Source: CAD feature listing. Evaluate the final solid. Frame: model axes, mm. Face numbers are marked on the shaded views. A direction names the side the tool comes from. Give positions to 0.01 mm unless a question says otherwise; leave off trailing zeros. Order: outer loops, then holes, each group sorted by start corner. A loop starts at its lowest first (then second) coordinate and runs counter-clockwise, first axis right, second up. Notation, with made-up numbers: M 66,63.5 L 116,63.5 A14 cw 116,67.5 Z; hole C 72.5,75.25 d8. An arc over 180 degrees is marked long. Answer in a Markdown table with one row per item. Add a question column.
(1) Section query B-B, the plane y = 7. Return loops of the section in (x, z) (3 decimals).
(2) Set-up query: the marked faces 1 and 2. Return all of +Z, -Z, +X, -X, +Y, -Y with unobstructed straight access to the full face (end or side cutting, diameter ignored); none if empty.
(3) Section query D-D, the plane x = -7. Return loops of the section in (y, z).
(4) Material intervals for line 1 along Y through (x, z) = (21.5, 10.5); line 2 along X through (y, z) = (2.5, 15); line 3 along X through (y, z) = (-22.5, 20.75), sorted ascending.
(5) Section query A-A, the plane z = 16.5. Return loops of the section in (x, y), plus the area to 3 significant figures.
(6) Mould query, pull axis Y, two halves, no side actions, for the marked faces 3, 4 and 5. Classes: pulls with the +Y half, pulls with the -Y half, needs draft (parallel to the pull), parting line crosses it, or undercut.
(7) Section query C-C, the plane z = 9.5. Return loops of the section in (x, y).
(8) Pin query (flat end, axial travel): P1, Ø3, axis at x = 27, y = -17, coming from the +Z side; P2, Ø3.5, axis at x = 33.25, y = 23.25, coming from the +Z side; P3, Ø1.2, axis at x = 36, z = 8, coming from the +Y side; P4, Ø2.5, axis at x = 27.4, y = 17.4, coming from the +Z side. Return the tip coordinate at first contact, or that it passes through.
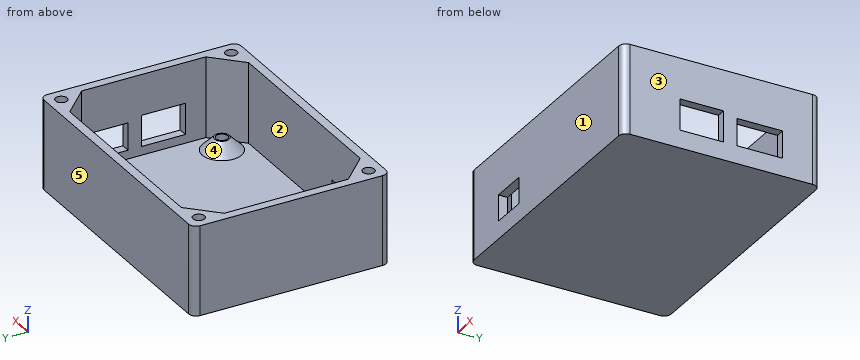
from build123d import *

# Parameters (mm, degrees)
SKETCH5_W           = 74
SKETCH5_H           = 54
BOSS_EXTRUDE4_DEPTH = 24.5
SHELL1_T            = -2.5
SKETCH6_R           = 2
BOSS_EXTRUDE5_DEPTH = 3.4
SKETCH11_R          = 1.6
CUT_EXTRUDE2_DEPTH  = 4.5
CUT_EXTRUDE4_REACH  = 84.494
SKETCH12_W          = 7.45
SKETCH12_H          = 12.5
CUT_EXTRUDE5_REACH  = 84.494
SKETCH13_W          = 8.5
SKETCH13_H          = 12
CUT_EXTRUDE6_REACH  = 71.895
SKETCH14_W          = 10
SKETCH14_H          = 7.138154435
BOSS_EXTRUDE7_DEPTH = 22
SKETCH9_R           = 1.6
CUT_EXTRUDE1_DEPTH  = 6.1
CHAMFER10_SIZE      = 3.4
CHAMFER11_SIZE      = 3.4
FILLET1_R           = 2


with BuildPart() as part:
    # Sketch5 → Boss-Extrude4 (new body)
    with BuildSketch(Plane.XY):
        Rectangle(SKETCH5_W, SKETCH5_H)
    extrude(amount=BOSS_EXTRUDE4_DEPTH)

    # Shell1
    shell1_openings = [part.faces().sort_by_distance(p)[0] for p in [
        (0, 0, 24.5),
    ]]
    offset(amount=SHELL1_T, openings=shell1_openings, kind=Kind.INTERSECTION)

    # Sketch6 → Boss-Extrude5 (add)
    with BuildSketch(Plane.XY.offset(2.5)):
        with Locations((-27.4, 17.4)):
            Circle(SKETCH6_R)
        with Locations((27.4, 17.4)):
            Circle(SKETCH6_R)
        with Locations((27.4, -17.4)):
            Circle(SKETCH6_R)
        with Locations((-27.4, -17.4)):
            Circle(SKETCH6_R)
    extrude(amount=BOSS_EXTRUDE5_DEPTH)

    # Sketch11 → Cut-Extrude2 (cut)
    with BuildSketch(Plane.XY.offset(5.9)):
        with Locations((-27.4, 17.4)):
            Circle(SKETCH11_R)
        with Locations((27.4, 17.4)):
            Circle(SKETCH11_R)
        with Locations((-27.4, -17.4)):
            Circle(SKETCH11_R)
        with Locations((27.4, -17.4)):
            Circle(SKETCH11_R)
    extrude(amount=-CUT_EXTRUDE2_DEPTH, mode=Mode.SUBTRACT)

    # Sketch12 → Cut-Extrude4 (cut, up to next)
    with BuildSketch(Plane(origin=(37, 0, 0), x_dir=(0, 0, -1), z_dir=(1, 0, 0)), mode=Mode.PRIVATE) as cut_extrude4_sk1:
        with Locations((-8.6, 10.53)):
            Rectangle(SKETCH12_W, SKETCH12_H)
    cut_extrude4_tool1 = extrude(cut_extrude4_sk1.sketch, amount=-CUT_EXTRUDE4_REACH, mode=Mode.PRIVATE) & part.part
    add(cut_extrude4_tool1.solids().sort_by_distance((37, 10.53, 8.6))[0], mode=Mode.SUBTRACT)

    # Sketch13 → Cut-Extrude5 (cut, up to next)
    with BuildSketch(Plane(origin=(37, 0, 0), x_dir=(0, 0, -1), z_dir=(1, 0, 0)), mode=Mode.PRIVATE) as cut_extrude5_sk1:
        with Locations((-9.125, -5.4)):
            Rectangle(SKETCH13_W, SKETCH13_H)
    cut_extrude5_tool1 = extrude(cut_extrude5_sk1.sketch, amount=-CUT_EXTRUDE5_REACH, mode=Mode.PRIVATE) & part.part
    add(cut_extrude5_tool1.solids().sort_by_distance((37, -5.4, 9.125))[0], mode=Mode.SUBTRACT)

    # Sketch14 → Cut-Extrude6 (cut, up to next)
    with BuildSketch(Plane.XZ.offset(27), mode=Mode.PRIVATE) as cut_extrude6_sk1:
        with Locations((-18.22, 8.449077218)):
            Rectangle(SKETCH14_W, SKETCH14_H)
    cut_extrude6_tool1 = extrude(cut_extrude6_sk1.sketch, amount=-CUT_EXTRUDE6_REACH, mode=Mode.PRIVATE) & part.part
    add(cut_extrude6_tool1.solids().sort_by_distance((-18.22, -27, 8.449077))[0], mode=Mode.SUBTRACT)

    # Sketch7 → Boss-Extrude7 (add)
    with BuildSketch(Plane.XY.offset(2.5)):
        Polygon((-27, 24.5), (-34.5, 17), (-34.5, 24.5), align=None)
        Polygon((-34.5, -17), (-27, -24.5), (-34.5, -24.5), align=None)
        Polygon((27, -24.5), (34.5, -17), (34.5, -24.5), align=None)
        Polygon((34.5, 17), (27, 24.5), (34.5, 24.5), align=None)
    extrude(amount=BOSS_EXTRUDE7_DEPTH)

    # Sketch9 → Cut-Extrude1 (cut)
    with BuildSketch(Plane.XY.offset(24.5)):
        with Locations((-33.25, 23.25)):
            Circle(SKETCH9_R)
        with Locations((33.25, 23.25)):
            Circle(SKETCH9_R)
        with Locations((-33.25, -23.25)):
            Circle(SKETCH9_R)
        with Locations((33.25, -23.25)):
            Circle(SKETCH9_R)
    extrude(amount=-CUT_EXTRUDE1_DEPTH, mode=Mode.SUBTRACT)

    # Chamfer10
    # the kernel refuses this chamfer: 3.4 mm, written as the material it adds along each edge
    with BuildSketch(Plane(origin=(-27.4, 17.4, 2.5), x_dir=(1, 0, 0), z_dir=(0, -1, 0))) as chamfer10_piece_1_section:
        Polygon((2 + CHAMFER10_SIZE, 0), (2, CHAMFER10_SIZE), (2, 0), align=None)
    chamfer10_piece_1 = revolve(axis=Axis((-27.4, 17.4, 2.5), (0, 0, 1)), mode=Mode.PRIVATE)
    chamfer10_piece_1 = split(chamfer10_piece_1, bisect_by=Plane(origin=(-31.112764442, 17.4, 5.9), z_dir=(0, 0, -1)), keep=Keep.TOP, mode=Mode.PRIVATE)
    add(chamfer10_piece_1)

    # Chamfer11
    # the kernel refuses this chamfer: 3.4 mm, written as the material it adds along each edge
    with BuildSketch(Plane(origin=(27.4, 17.4, 2.5), x_dir=(1, 0, 0), z_dir=(0, -1, 0))) as chamfer11_piece_1_section:
        Polygon((2 + CHAMFER11_SIZE, 0), (2, CHAMFER11_SIZE), (2, 0), align=None)
    chamfer11_piece_1 = revolve(axis=Axis((27.4, 17.4, 2.5), (0, 0, 1)), mode=Mode.PRIVATE)
    chamfer11_piece_1 = split(chamfer11_piece_1, bisect_by=Plane(origin=(23.687235558, 17.4, 5.9), z_dir=(0, 0, -1)), keep=Keep.TOP, mode=Mode.PRIVATE)
    add(chamfer11_piece_1)
    with BuildSketch(Plane(origin=(27.4, -17.4, 2.5), x_dir=(1, 0, 0), z_dir=(0, -1, 0))) as chamfer11_piece_2_section:
        Polygon((2 + CHAMFER11_SIZE, 0), (2, CHAMFER11_SIZE), (2, 0), align=None)
    chamfer11_piece_2 = revolve(axis=Axis((27.4, -17.4, 2.5), (0, 0, 1)), mode=Mode.PRIVATE)
    chamfer11_piece_2 = split(chamfer11_piece_2, bisect_by=Plane(origin=(23.687235558, -17.4, 5.9), z_dir=(0, 0, -1)), keep=Keep.TOP, mode=Mode.PRIVATE)
    add(chamfer11_piece_2)
    with BuildSketch(Plane(origin=(-27.4, -17.4, 2.5), x_dir=(1, 0, 0), z_dir=(0, -1, 0))) as chamfer11_piece_3_section:
        Polygon((2 + CHAMFER11_SIZE, 0), (2, CHAMFER11_SIZE), (2, 0), align=None)
    chamfer11_piece_3 = revolve(axis=Axis((-27.4, -17.4, 2.5), (0, 0, 1)), mode=Mode.PRIVATE)
    chamfer11_piece_3 = split(chamfer11_piece_3, bisect_by=Plane(origin=(-31.112764442, -17.4, 5.9), z_dir=(0, 0, -1)), keep=Keep.TOP, mode=Mode.PRIVATE)
    add(chamfer11_piece_3)

    # Fillet1
    fillet1_edges = [part.edges().sort_by_distance(p)[0] for p in [
        (37, -27, 12.25),
        (-37, -27, 12.25),
        (-37, 27, 12.25),
        (37, 27, 12.25),
    ]]
    fillet(fillet1_edges, radius=FILLET1_R)


solid = part.part
Values follow:
| question | item | result |
|---|---|---|
| 1 | outline | M -37,0 L 37,0 L 37,4.875 L 34.5,4.875 L 34.5,2.5 L -34.5,2.5 L -34.5,24.5 L -37,24.5 Z; M 34.5,12.325 L 37,12.325 L 37,24.5 L 34.5,24.5 Z |
| 2 | face 1 | +Z, -Z, +X, -X, -Y |
| 2 | face 2 | +Z |
| 3 | outline | M -27,0 L 27,0 L 27,24.5 L 24.5,24.5 L 24.5,2.5 L -24.5,2.5 L -24.5,24.5 L -27,24.5 Z |
| 4 | line 1 | y = -27 to -24.5, 24.5 to 27 |
| 4 | line 2 | x = -37 to -34.5, 34.5 to 37 |
| 4 | line 3 | x = -37 to -34.66, -31.84 to -29, 29 to 31.84, 34.66 to 37 |
| 5 | outline | M -37,-25 A2 ccw -35,-27 L 35,-27 A2 ccw 37,-25 L 37,25 A2 ccw 35,27 L -35,27 A2 ccw -37,25 Z; hole M -34.5,-17 L -27,-24.5 L 27,-24.5 L 34.5,-17 L 34.5,17 L 27,24.5 L -27,24.5 L -34.5,17 Z |
| 5 | area | 724 mm² |
| 6 | face 3 | needs draft |
| 6 | face 4 | undercut |
| 6 | face 5 | pulls with the +Y half |
| 7 | outline | M -37,-25 A2 ccw -35,-27 L -23.22,-27 L -23.22,-24.5 L -27,-24.5 L -34.5,-17 L -34.5,17 L -27,24.5 L 27,24.5 L 34.5,17 L 34.5,16.78 L 37,16.78 L 37,25 A2 ccw 35,27 L -35,27 A2 ccw -37,25 Z; M -13.22,-27 L 35,-27 A2 ccw 37,-25 L 37,-11.4 L 34.5,-11.4 L 34.5,-17 L 27,-24.5 L -13.22,-24.5 Z; M 34.5,0.6 L 37,0.6 L 37,4.28 L 34.5,4.28 Z |
| 8 | P1 | stops at z = 5.9 |
| 8 | P2 | stops at z = 24.5 |
| 8 | P3 | stops at y = 26.96 |
| 8 | P4 | stops at z = 1.4 |
